Source: CAD feature listing. Evaluate the final solid. Frame: model axes, mm. Give positions to 0.01 mm unless a question says otherwise; leave off trailing zeros. Write each loop counter-clockwise with the first axis right and the second up, starting at its lowest first coordinate (ties: lowest second). Pieces come first, ordered by that corner, then holes. Notation, with made-up numbers: (59, 35.5) -> (100, 35.5) arc R21 ccw to (100, 61.5) -> close; hole circle Ø4 at (1.25, -14). An arc over 180 degrees is marked (long way). Use one line per item in the form item = value. Start each with the question number.
(1) Cut plane B-B, the plane x = 29. Output: boundary loops of the cut face in (y, z).
(2) Material intervals for line 1 along X through (y, z) = (0.75, 0); line 2 along X through (y, z) = (3.05, -5.75); line 3 along Z through (x, y) = (33, 0.45), sorted ascending. Write a range as from..to.
(3) Cut plane A-A, the plane z = -5. Output: boundary loops of the cut face in (x, y).
(4) Cut plane D-D, the plane z = 5.25. Output: boundary loops of the cut face in (x, y), and give its area (3 significant figures).
(5) Cut plane C-C, the plane y = 2.6. Output: boundary loops of the cut face in (x, z), and give its area (3 significant figures).
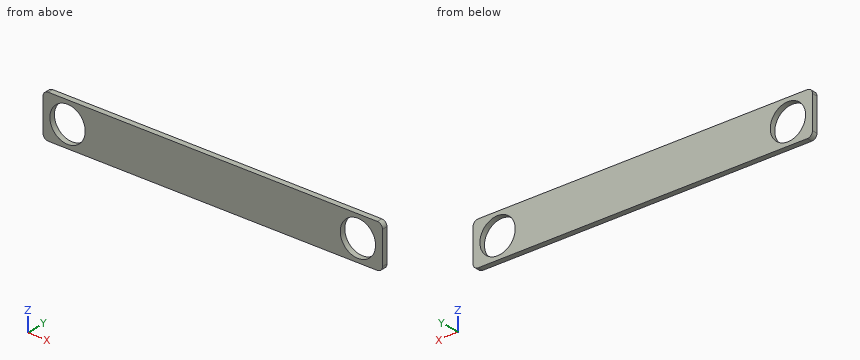
from build123d import *

# Parameters (mm, degrees)
SKETCH1_W           = 197
SKETCH1_H           = 25
SKETCH1_R           = 10.25
BOSS_EXTRUDE1_DEPTH = 3.2
FILLET1_R           = 3


with BuildPart() as part:
    # Sketch1 → Boss-Extrude1 (new body)
    with BuildSketch(Plane(origin=(0, 0, 0), x_dir=(1, 0, 0), z_dir=(0, 1, 0))):
        with Locations((-53.132, 0)):
            Rectangle(SKETCH1_W, SKETCH1_H)
        with Locations(Location((31.118, 0, 0), (0, 0, 270))):
            Circle(SKETCH1_R, mode=Mode.SUBTRACT)
        with Locations(Location((-137.382, 0, 0), (0, 0, 270))):
            Circle(SKETCH1_R, mode=Mode.SUBTRACT)
    extrude(amount=BOSS_EXTRUDE1_DEPTH)

    # Fillet1
    fillet1_edges = [part.edges().sort_by_distance(p)[0] for p in [
        (45.368, 1.6, -12.5),
        (45.368, 1.6, 12.5),
        (-151.632, 1.6, 12.5),
        (-151.632, 1.6, -12.5),
    ]]
    fillet(fillet1_edges, radius=FILLET1_R)


solid = part.part
Geometry says:
q1.outline = (0, -12.5) -> (3.2, -12.5) -> (3.2, -10.03) -> (0, -10.03) -> close; (0, 10.03) -> (3.2, 10.03) -> (3.2, 12.5) -> (0, 12.5) -> close
q2.line_1 = -151.63..-147.63, -127.13..20.87, 41.37..45.37
q2.line_2 = -151.63..-145.87, -128.9..22.63, 39.6..45.37
q2.line_3 = -12.5..-10.08, 10.08..12.5
q3.outline = (-151.63, 0) -> (-146.33, 0) -> (-146.33, 3.2) -> (-151.63, 3.2) -> close; (-128.43, 0) -> (22.17, 0) -> (22.17, 3.2) -> (-128.43, 3.2) -> close; (40.07, 0) -> (45.37, 0) -> (45.37, 3.2) -> (40.07, 3.2) -> close
q4.outline = (-151.63, 0) -> (-146.19, 0) -> (-146.19, 3.2) -> (-151.63, 3.2) -> close; (-128.58, 0) -> (22.31, 0) -> (22.31, 3.2) -> (-128.58, 3.2) -> close; (39.92, 0) -> (45.37, 0) -> (45.37, 3.2) -> (39.92, 3.2) -> close
q4.area = 518 mm^2
q5.outline = (-151.63, -9.5) arc R3 ccw to (-148.63, -12.5) -> (42.37, -12.5) arc R3 ccw to (45.37, -9.5) -> (45.37, 9.5) arc R3 ccw to (42.37, 12.5) -> (-148.63, 12.5) arc R3 ccw to (-151.63, 9.5) -> close; hole circle Ø20.5 at (-137.38, 0); hole circle Ø20.5 at (31.12, 0)
q5.area = 4,260 mm^2
